Input: part model. Units: mm. Frame: model coordinates. A direction names the side the tool comes from. Coordinates: 2 decimals unless noted, no trailing zeros. Order: outer loops, then holes, each group sorted by start corner. A loop starts at its lowest first (then second) coordinate and runs counter-clockwise, first axis right, second up.
from build123d import *

# Parameters (mm, degrees)
BOSS_EXTRUDE1_DEPTH         = 3.175
F_1_4_0_25_DIAMETER_HOLE1_D = 6.35
F_1_4_0_25_DIAMETER_HOLE2_D = 6.35


with BuildPart() as part:
    # Sketch2 → Boss-Extrude1 (new body)
    with BuildSketch(Plane(origin=(0, 0, 0), x_dir=(1, 0, 0), z_dir=(0, 1, 0))):
        with BuildLine():
            Line((-431.938028743, -442.700646237), (-335.418028743, -442.700646237))
            ThreePointArc((-335.418028743, -442.700646237), (-333.621977519, -441.956697461), (-332.878028743, -440.160646237))
            Line((-332.878028743, -440.160646237), (-332.878028743, -419.840646237))
            ThreePointArc((-332.878028743, -419.840646237), (-333.621977519, -418.044595013), (-335.418028743, -417.300646237))
            Line((-335.418028743, -417.300646237), (-370.978028743, -417.300646237))
            ThreePointArc((-370.978028743, -417.300646237), (-397.918797106, -406.1414146), (-409.078028743, -379.200646237))
            Line((-409.078028743, -379.200646237), (-409.078028743, -343.640646237))
            ThreePointArc((-409.078028743, -343.640646237), (-409.821977519, -341.844595013), (-411.618028743, -341.100646237))
            Line((-411.618028743, -341.100646237), (-431.938028743, -341.100646237))
            ThreePointArc((-431.938028743, -341.100646237), (-433.734079967, -341.844595013), (-434.478028743, -343.640646237))
            Line((-434.478028743, -343.640646237), (-434.478028743, -440.160646237))
            ThreePointArc((-434.478028743, -440.160646237), (-433.734079967, -441.956697461), (-431.938028743, -442.700646237))
        make_face()
    extrude(amount=BOSS_EXTRUDE1_DEPTH)

    # 1/4 (0.25) Diameter Hole1 (through all)
    with Locations(Plane(origin=(0, 3.175, 0), x_dir=(1, 0, 0), z_dir=(0, 1, 0))):
        with Locations((-421.778028743, -353.800646237), (-421.778028743, -379.200646237), (-370.978028743, -430.000646237), (-345.578028743, -430.000646237)):
            Hole(F_1_4_0_25_DIAMETER_HOLE1_D / 2)

    # 1/4 (0.25) Diameter Hole2 (through all)
    with Locations(Plane(origin=(0, 3.175, 0), x_dir=(1, 0, 0), z_dir=(0, 1, 0))):
        with Locations((-421.778028743, -430.000646237), (-396.378028743, -430.000646237), (-421.778028743, -404.600646237)):
            Hole(F_1_4_0_25_DIAMETER_HOLE2_D / 2)


solid = part.part
Item 1: Cut plane A-A on x = -396. Return loops of the section in (y, z) (3 decimals), then the cut area to 3 significant figures.
Response values:
outline: (0, 407.932) - (3.175, 407.932) - (3.175, 426.848) - (0, 426.848) - close; (0, 433.153) - (3.175, 433.153) - (3.175, 442.701) - (0, 442.701) - close
area: 90.4 mm2
Item 2: Draft query along X for faces 1 (the face through (-373.91, 1.57, 431.22)), 2 (the face through (-409.802, 1.565, 341.864)), 3 (the face through (-384, 2, 442.701)). Return one class per face: pulls with the +X half, pulls with the -X half, needs draft (parallel to the pull), parting line crosses it, or undercut.
Response values:
face 1: undercut
face 2: pulls with the +X half
face 3: needs draft
Item 3: Cut plane C-C on z = 374.5. Return loops of the section in (x, y) (3 decimals).
Response values:
outline: (-434.478, 0) - (-409.078, 0) - (-409.078, 3.175) - (-434.478, 3.175) - close
Item 4: Access query for faces 4 (the face through (-422, 2, 341.101)), 5 (the face through (-353, 2, 417.301)). Directions: +Z, -Z, +X, -X, +Y, -Y. A direction counts if a zero-diameter tool reaches every point of the face in a straight line with its end or side. Return the directions, or none.
Response values:
face 4: -Z, +X, -X, +Y, -Y
face 5: -Z, +X, +Y, -Y
Item 5: Ray query, probe 1 along Z at (x, y) = (-371, 2.95); probe 2 along Z at (x, y) = (-422.5, 0.35); probe 3 along Z at (x, y) = (-372.5, 1.05). Return the intervals inside material, ascending.
Response values:
probe 1: z = 417.3 to 426.83, 433.18 to 442.7
probe 2: z = 341.1 to 350.71, 356.89 to 376.11, 382.29 to 401.51, 407.69 to 426.91, 433.09 to 442.7
probe 3: z = 417.27 to 427.21, 432.79 to 442.7
Item 6: Cut plane B-B on y = 2.1. Return loops of the section in (x, z) (3 decimals).
Response values:
outline: (-434.478, 343.641) arc R2.54 ccw to (-431.938, 341.101) - (-411.618, 341.101) arc R2.54 ccw to (-409.078, 343.641) - (-409.078, 379.201) arc R38.1 cw to (-370.978, 417.301) - (-335.418, 417.301) arc R2.54 ccw to (-332.878, 419.841) - (-332.878, 440.161) arc R2.54 ccw to (-335.418, 442.701) - (-431.938, 442.701) arc R2.54 ccw to (-434.478, 440.161) - close; hole circle Ø6.35 at (-421.778, 353.801); hole circle Ø6.35 at (-421.778, 379.201); hole circle Ø6.35 at (-421.778, 404.601); hole circle Ø6.35 at (-421.778, 430.001); hole circle Ø6.35 at (-396.378, 430.001); hole circle Ø6.35 at (-370.978, 430.001); hole circle Ø6.35 at (-345.578, 430.001)
Item 7: Pin query (flat end, axial travel): pin 1 Ø1 at (y, z) = (2.5, 385) entering from +X. Return the tip coordinate at first contact, or that it passes through.
Response values:
pin 1: stops at x = -408.55
Item 8: Cut plane D-D on x = -365. Return loops of the section in (y, z) (3 decimals).
Response values:
outline: (0, 417.301) - (3.175, 417.301) - (3.175, 442.701) - (0, 442.701) - close
